Autodesk Inventor part; units mm, degrees
ref_plane "YZ Plane" through (0, 0, 0) normal (1, 0, 0) x (0, 1, 0)
ref_plane "XZ Plane" through (0, 0, 0) normal (0, 1, 0) x (-1, 0, 0)
ref_plane "XY Plane" through (0, 0, 0) normal (0, 0, 1) x (1, 0, 0)
sketch "Sketch1" plane through (0, 0, 0) normal (0, 0, 1) x (1, 0, 0)
  line L0 (0, 0) -> (195.58, 0)
  line L1 (195.58, 0) -> (195.58, 50.8)
  line L2 (195.58, 50.8) -> (0, 50.8)
  line L3 (0, 50.8) -> (0, 0)
  dimension "d0" = 195.58
  dimension "d1" = 50.8
extrude "Extrusion1" add sketch "Sketch1" along normal blind 0.762
sketch "Sketch2" plane through (0, 0, 0.762) normal (0, 0, 1) x (1, 0, 0)
  circle A0 centre (4.7625, 4.7625) radius 2.2479
  circle A1 centre (78.4225, 4.7625) radius 2.2479
  circle A2 centre (117.1575, 4.7625) radius 2.2479
  circle A3 centre (190.8175, 4.7625) radius 2.2479
hole "Hole1" at (4.7625, 4.7625, 0.762) at (78.4225, 4.7625, 0.762) at (117.1575, 4.7625, 0.762) at (190.8175, 4.7625, 0.762) direction (0, 0, -1) diameter 4.318 end through all
sketch "Sketch3" plane through (0, 0, 0.762) normal (0, 0, 1) x (1, 0, 0)
  line L0 (195.58, 0) -> (0, 0)
  point P0 (4.7625, 25.4)
  point P1 (78.4225, 15.24)
  point P2 (117.1575, 15.24)
  point P3 (190.8175, 25.4)
  dimension "d11" = 25.4
  dimension "d12" = 15.24
  dimension "d13" = 15.24
  dimension "d14" = 25.4
hole "Hole2" at (4.7625, 25.4, 0.762) at (78.4225, 15.24, 0.762) at (117.1575, 15.24, 0.762) at (190.8175, 25.4, 0.762) direction (0, 0, -1) diameter 4.318 end through all
properties part number "Blade" material "Steel"
Verification items for the finished model (mm, model axes). Coordinates: 2 decimals unless noted, no trailing zeros. Write each loop counter-clockwise with the first axis right and the second up, starting at its lowest first coordinate (ties: lowest second). Pieces come first, ordered by that corner, then holes. Notation, with made-up numbers: (-38, 36.5) - (-6, 36.5) arc R17 cw to (-6, 49.5) - close; hole circle Ø9 at (74, 72.5). An arc over 180 degrees is marked (long way). One line per question, with ' | ' between items. Start each with the question number.
1. Section check A-A (y = 15.24). Enter the section's corners in (x, z), plus the area to 3 significant figures.
2. Gauge pin test, flat end, axial feed: P1, Ø2.5, axis at x = 117.16, y = 15.24, coming from the -Z side. Record the tip position at first contact, or that the pin passes through.
3. Material ranges on line 1 along X through (y, z) = (25.4, 0.4); line 2 along X through (y, z) = (14, 0.55), recorded low to high.
4. Draft check along Y on faces 1 (the cylindrical face through (76.602, 3.602, 0.376)), 2 (the flat face through (96, 26, 0)). Enter one of: released by +Y, released by -Y, zero draft, split by the parting line, or undercut.
Computed values:
1) outline: (0, 0) - (76.26, 0) - (76.26, 0.76) - (0, 0.76) - close; (80.58, 0) - (115, 0) - (115, 0.76) - (80.58, 0.76) - close; (119.32, 0) - (195.58, 0) - (195.58, 0.76) - (119.32, 0.76) - close | area: 142 mm²
2) P1: through
3) line 1: 0 to 2.6, 6.92 to 188.66, 192.98 to 195.58 | line 2: 0 to 76.66, 80.19 to 115.39, 118.92 to 195.58
4) face 1: undercut | face 2: zero draft
